The listing builds one solid part. Answer for the finished solid, in the listing's coordinates (mm). A direction names the side the tool comes from. Round coordinates to 2 decimals unless told otherwise and drop trailing zeros. Write each loop counter-clockwise with the first axis right and the second up, starting at its lowest first coordinate (ties: lowest second). Pieces come first, ordered by that corner, then holes.
from build123d import *

# Parameters (mm, degrees)
F3_DEPTH       = 5.001
F4_W           = 0.7
F4_H           = 2.9
F5_ANGLE_BACK  = 17.589911292
F5_ANGLE       = 77.589911292
F6_W           = 0.7
F6_H           = 7.3
F7_ANGLE_START = 300
F7_ANGLE       = 28
F8_SIZE        = 0.4
F9_R           = 0.4


with BuildPart() as f1:
    # F0 (on Front) → F1 (revolve)
    with BuildSketch(Plane.XZ):
        Polygon((-13.05, 15.0180591579), (-7.8, 15.0180591579), (-7.8, 25.6180591579), (-9.2, 25.6180591579), (-9.2, 16.4180591579), (-11.65, 16.4180591579), (-11.65, 20.0180591579), (-16.875, 20.0180591579), (-16.875, 18.6180591579), (-13.05, 18.6180591579), align=None)
    revolve(axis=Axis((0, 0, 52.8953172941), (0, 0, 1)))

    # F2 (on face) → F3 (cut, through all)
    with BuildSketch(Plane.XY.offset(20.0180591579)):
        with BuildLine():
            Line((-4, 13.05), (-4, 16.3940728619))
            ThreePointArc((-4, 16.3940728619), (-7.5371728948, 15.0982333322), (-10.6987440852, 13.05))
            Line((-10.6987440852, 13.05), (-4, 13.05))
        make_face()
        with BuildLine():
            ThreePointArc((10.6987440852, 13.05), (7.5371728948, 15.0982333322), (4, 16.3940728619))
            Line((4, 16.3940728619), (4, 13.05))
            Line((4, 13.05), (10.6987440852, 13.05))
        make_face()
        with BuildLine():
            ThreePointArc((4, 16.3940728619), (0, 16.875), (-4, 16.3940728619))
            Line((-4, 16.3940728619), (4, 16.3940728619))
        make_face()
    extrude(amount=-F3_DEPTH, mode=Mode.SUBTRACT)

    # F4 (on Right) → F5 (revolve, cut)
    with BuildSketch(Plane.YZ, mode=Mode.PRIVATE) as f5_sk:
        with Locations((8.15, 19.7680591579)):
            Rectangle(F4_W, F4_H)
        with Locations((-8.15, 19.7680591579)):
            Rectangle(F4_W, F4_H)
    revolve(f5_sk.sketch.rotate(Axis((0, 0, 20.0180591579), (0, 0, 1)), -F5_ANGLE_BACK), axis=Axis((0, 0, 20.0180591579), (0, 0, 1)), revolution_arc=F5_ANGLE, mode=Mode.SUBTRACT)

    # F6 (on Right) → F7 (revolve, cut)
    with BuildSketch(Plane.YZ, mode=Mode.PRIVATE) as f7_sk:
        with Locations((8.15, 21.9680591579)):
            Rectangle(F6_W, F6_H)
        with Locations((-8.15, 21.9680591579)):
            Rectangle(F6_W, F6_H)
    revolve(f7_sk.sketch.rotate(Axis((0, 0, 15.0180591579), (0, 0, -1)), F7_ANGLE_START), axis=Axis((0, 0, 15.0180591579), (0, 0, -1)), revolution_arc=F7_ANGLE, mode=Mode.SUBTRACT)

    # F8
    f8_edges = [f1.edges().sort_by_distance(p)[0] for p in [
        (5.418335, 5.61085, 25.618059),
        (-7.534221, 2.018789, 25.618059),
    ]]
    chamfer(f8_edges, length=F8_SIZE)

    # F9
    f9_edges = [f1.edges().sort_by_distance(p)[0] for p in [
        (13.05, 0, 15.018059),
    ]]
    fillet(f9_edges, radius=F9_R)


solid = f1.part
1. Section C-C on z = 23 is taken. Determine the outline of the cut face in (x, y) (3 decimals).
Geometry says:
outline: circle Ø18.4 at (0, 0); hole (-7.361, 4.25) - (-6.755, 3.9) arc R7.8 ccw to (4.133, -6.615) - (4.504, -7.208) arc R8.5 ccw to (7.361, -4.25) - (6.755, -3.9) arc R7.8 ccw to (-4.133, 6.615) - (-4.504, 7.208) arc R8.5 ccw to start
2. For a pull along Y with two mould halves and no side action, classify faces 1 (the face through (-0.58, -16.865, 19.308)), 2 (the face through (1, -8, 21.218)), 3 (the face through (-7, 13.05, 19)) as released by +Y, released by -Y, zero draft, split by the parting line, or undercut.
Geometry says:
face 1: split by the parting line
face 2: undercut
face 3: released by +Y
3. Straight lines are drawn through the part: line 1 along Y through (x, z) = (0, 18.9) (3 decimals); line 2 along X through (y, z) = (0, 19.2) (3 decimals); line 3 along X through (y, z) = (0, 18.5). For each, find the intervals that lie inside material, in ascending order.
Geometry says:
line 1: y = -16.875 to -11.65, -9.2 to -8.5, 8.5 to 9.2, 11.65 to 16.394
line 2: x = -16.875 to -11.65, -9.2 to -7.8, 7.8 to 9.2, 11.65 to 16.875
line 3: x = -13.05 to -11.65, -9.2 to -7.8, 7.8 to 9.2, 11.65 to 13.05
4. A tool of negligible diameter and unlimited length cuts with its end or side. For faces 4 (the face through (4.3, -7.33, 20.4)), 5 (the face through (-4, 15, 19)), 6 (the face through (7, 13.05, 19)), 7 (the face through (7.3, 5.6, 21)), 8 (the face through (-4, -13, 18.618)), from which of +Z, -Z, +X, -X, +Y, -Y can it reach the whole face along a straight path? Write none if from no direction.
Geometry says:
face 4: none
face 5: +Z, -Z, -X, +Y
face 6: +Z, -Z, +X, +Y
face 7: +Z
face 8: -Z
5. Section D-D on z = 17.5 is taken. Determine the outline of the cut face in (x, y).
Geometry says:
outline: circle Ø26.1 at (0, 0); circle Ø18.4 at (0, 0); hole circle Ø23.3 at (0, 0); hole circle Ø15.6 at (0, 0)
6. Given pin 1 (4 mm diameter, centred on x = -10, z = 18, fed in from -Y); pin 2 (1.5 mm diameter, centred on x = 10.5, z = 24.5, fed in from -Y); pin 3 (1.1 mm diameter, centred on y = 14.5, z = 19, fed in from +X); pin 4 (1.5 mm diameter, centred on y = 14.5, z = 19.5, fed in from -X), each flat-ended and moving along its own axis, determine where each tip first touches the part or whether it passes through.
Geometry says:
pin 1: stops at y = -14.81
pin 2: passes through
pin 3: stops at x = 4
pin 4: stops at x = -4
7. Section A-A on y = 0 is taken. Determine the outline of the cut face in (x, z) (3 decimals).
Geometry says:
outline: (-16.875, 18.618) - (-13.05, 18.618) - (-13.05, 15.418) arc R0.4 ccw to (-12.65, 15.018) - (-7.8, 15.018) - (-7.8, 25.218) - (-8.2, 25.618) - (-9.2, 25.618) - (-9.2, 16.418) - (-11.65, 16.418) - (-11.65, 20.018) - (-16.875, 20.018) - close; (7.8, 15.018) - (12.65, 15.018) arc R0.4 ccw to (13.05, 15.418) - (13.05, 18.618) - (16.875, 18.618) - (16.875, 20.018) - (11.65, 20.018) - (11.65, 16.418) - (9.2, 16.418) - (9.2, 25.618) - (8.2, 25.618) - (7.8, 25.218) - close
